Input: part model. Units: mm. Frame: model coordinates. A direction names the side the tool comes from. Round coordinates to 2 decimals unless told otherwise and drop trailing zeros. Loops run counter-clockwise (first coordinate to the right, second up) from the corner with the lowest first, then second, coordinate; pieces in that order, holes last. Notation, with made-up numbers: (-16, 63.25) -> (2, 63.25) arc R20 ccw to (2, 83.25) -> close; hole circle Ø4 at (48, -17). An arc over 180 degrees is marked (long way). Answer in a Markdown table with one row per item. Add a question column.
Q1. Mould query, pull axis Y, two halves, no side actions, for faces 5 (the face through (15, 0, 0)), 6 (the face through (0, -15, 0)), 7 (the face through (7.85, -8, 7)). Classes: pulls with the +Y half, pulls with the -Y half, needs draft (parallel to the pull), parting line crosses it, or undercut.
Q2. Section C-C, the plane z = -12. Output: boundary loops of the cut face in (x, y), and give its area (3 significant figures).
Q3. Section A-A, the plane x = -7.5. Output: boundary loops of the cut face in (y, z), and give its area (3 significant figures).
Q4. Section B-B, the plane z = 5.5. Output: boundary loops of the cut face in (x, y), and give its area (3 significant figures).
Q5. Reachability of faces 1 (the face through (-7.708, 8.887, -7.395)), 2 (the face through (-12, 0, 0)), 3 (the face through (2.2, 0, 7)), 4 (the face through (-9.798, 2.093, 7.395)) from +Z, -Z, +X, -X, +Y, -Y: full face, straight path, thin tool, end or side. Return the list, or none.
Q6. Ray query, L1, parallel to Y at x = -7.5, z = 6; L2, parallel to X at y = -6.5, z = 4; L3, parallel to Y at x = -7.5, z = -6.5. Return the intervals inside material, ascending. Write a range as from..to.
Q7. Pin query (flat end, axial travel): pin 1 (5 mm diameter, centred on x = 5, y = 0, fed in from +Z). Return the tip coordinate at first contact, or that it passes through.
```python
from build123d import *

# Parameters (mm, degrees)
SKETCH_W        = 30
SKETCH_H        = 30
PAD_DEPTH       = 15
SKETCH001_R     = 1.6
SKETCH001_R_2   = 2.6
SKETCH001_R_3   = 3.1
POCKET_DEPTH    = 15.001
SKETCH002_R     = 1.25
SKETCH002_R_2   = 2.3
SKETCH002_R_3   = 2.75
POCKET001_DEPTH = 15.001
SKETCH003_W     = 10
SKETCH003_H     = 10
POCKET002_DEPTH = 3


with BuildPart() as part:
    # Sketch → Pad (new body, symmetric)
    with BuildSketch(Plane.XZ):
        Rectangle(SKETCH_W, SKETCH_H)
    extrude(amount=PAD_DEPTH, both=True)

    # Sketch001 → Pocket (cut, through all)
    with BuildSketch(Plane.XY):
        with Locations((-7.5, 7.300443)):
            Circle(SKETCH001_R)
        with Locations((-7.5, 1.991905)):
            Circle(SKETCH001_R_2)
        with Locations((-7.5, -5)):
            Circle(SKETCH001_R_3)
        with Locations((5, 7.5)):
            Circle(SKETCH001_R)
        with Locations((5, 0)):
            Circle(SKETCH001_R)
        with Locations((5, -7.5)):
            Circle(SKETCH001_R)
    extrude(amount=-POCKET_DEPTH, mode=Mode.SUBTRACT)

    # Sketch002 → Pocket001 (cut, through all)
    with BuildSketch(Plane.XY):
        with Locations((-7.5, 7.300443)):
            Circle(SKETCH002_R)
        with Locations((-7.5, 1.991905)):
            Circle(SKETCH002_R_2)
        with Locations((-7.5, -5)):
            Circle(SKETCH002_R_3)
        Polygon((7.75, 5.912287), (7.75, 9.087713), (5, 10.675426), (2.25, 9.087713), (2.25, 5.912287), (5, 4.324574), align=None)
        Polygon((7.8, -1.616581), (7.8, 1.616581), (5, 3.233162), (2.2, 1.616581), (2.2, -1.616581), (5, -3.233162), align=None)
        Polygon((7.85, -9.145448), (7.85, -5.854552), (5, -4.209103), (2.15, -5.854552), (2.15, -9.145448), (5, -10.790897), align=None)
    extrude(amount=POCKET001_DEPTH, mode=Mode.SUBTRACT)

    # Sketch003 (on Face2 of Pocket001) → Pocket002 (cut)
    with BuildSketch(Plane(origin=(-15, 0, 0), x_dir=(0, 0, -1), z_dir=(-1, 0, 0))):
        Rectangle(SKETCH003_W, SKETCH003_H)
    extrude(amount=-POCKET002_DEPTH, mode=Mode.SUBTRACT)


solid = part.part
```
Answer block:
| question | item | result |
|---|---|---|
| 1 | face 5 | needs draft |
| 1 | face 6 | pulls with the -Y half |
| 1 | face 7 | undercut |
| 2 | outline | (-15, -15) -> (15, -15) -> (15, 15) -> (-15, 15) -> close; hole circle Ø6.2 at (-7.5, -5); hole circle Ø5.2 at (-7.5, 1.99); hole circle Ø3.2 at (-7.5, 7.3); hole circle Ø3.2 at (5, -7.5); hole circle Ø3.2 at (5, 0); hole circle Ø3.2 at (5, 7.5) |
| 2 | area | 816 mm^2 |
| 3 | outline | (-15, -15) -> (-8.1, -15) -> (-8.1, 0) -> (-7.75, 0) -> (-7.75, 15) -> (-15, 15) -> close; (-2.25, 0) -> (-1.9, 0) -> (-1.9, -15) -> (-0.61, -15) -> (-0.61, 0) -> (-0.31, 0) -> (-0.31, 15) -> (-2.25, 15) -> close; (4.29, 0) -> (4.59, 0) -> (4.59, -15) -> (5.7, -15) -> (5.7, 0) -> (6.05, 0) -> (6.05, 15) -> (4.29, 15) -> close; (8.55, 0) -> (8.9, 0) -> (8.9, -15) -> (15, -15) -> (15, 15) -> (8.55, 15) -> close |
| 3 | area | 492 mm^2 |
| 4 | outline | (-15, -15) -> (15, -15) -> (15, 15) -> (-15, 15) -> close; hole circle Ø5.5 at (-7.5, -5); hole circle Ø4.6 at (-7.5, 1.99); hole circle Ø2.5 at (-7.5, 7.3); hole (2.15, -9.15) -> (5, -10.79) -> (7.85, -9.15) -> (7.85, -5.85) -> (5, -4.21) -> (2.15, -5.85) -> close; hole (2.2, -1.62) -> (5, -3.23) -> (7.8, -1.62) -> (7.8, 1.62) -> (5, 3.23) -> (2.2, 1.62) -> close; hole (2.25, 5.91) -> (5, 4.32) -> (7.75, 5.91) -> (7.75, 9.09) -> (5, 10.68) -> (2.25, 9.09) -> close |
| 4 | area | 773 mm^2 |
| 5 | face 1 | -Z |
| 5 | face 2 | -X |
| 5 | face 3 | +Z |
| 5 | face 4 | +Z, -Z |
| 6 | L1 | -15..-7.75, -2.25..-0.31, 4.29..6.05, 8.55..15 |
| 6 | L2 | -15..-9.8, -5.2..2.15, 7.85..15 |
| 6 | L3 | -15..-8.1, -1.9..-0.61, 4.59..5.7, 8.9..15 |
| 7 | pin 1 | z = 0 |
